Autodesk Inventor part; units mm, degrees
ref_plane "YZ Plane" through (0, 0, 0) normal (1, 0, 0) x (0, 1, 0)
ref_plane "XZ Plane" through (0, 0, 0) normal (0, 1, 0) x (-1, 0, 0)
ref_plane "XY Plane" through (0, 0, 0) normal (0, 0, 1) x (1, 0, 0)
sketch "Sketch1" plane through (0, 0, 0) normal (0, 1, 0) x (-1, 0, 0)
  line L0 (6.15, 6.15) -> (-6.15, 6.15)
  line L1 (-6.15, 6.15) -> (-6.15, -6.15)
  line L2 (-6.15, -6.15) -> (6.15, -6.15)
  line L3 (6.15, -6.15) -> (6.15, 6.15)
  point P0 (0, 0)
  dimension "d0" = 12.3
  dimension "d1" = 12.3
  dimension "d2" = 6.15
  dimension "d3" = 6.15
extrude "Extrusion1" add sketch "Sketch1" along normal blind 5.5
fillet "Fillet1" radius 3.175 4 edges at (6.15, 2.75, 6.15) (-6.15, 2.75, 6.15) (6.15, 2.75, -6.15) (-6.15, 2.75, -6.15)
sketch "Sketch2" plane through (0, 5.5, 0) normal (0, 1, 0) x (1, 0, 0)
  circle A0 centre (0, 0) radius 4.9967
extrude "Extrusion2" add sketch "Sketch2" along normal blind 0.5
chamfer "Chamfer1" distance 1 angle 45 8 edges at (0, 0, 6.15) (5.2201, 0, 5.2201) (6.15, 0, 0) (5.2201, 0, -5.2201) (0, 0, -6.15) (-5.2201, 0, -5.2201) (-6.15, 0, 0) (-5.2201, 0, 5.2201)
sketch "Sketch3" plane through (0, 0, 0) normal (0, -1, 0) x (1, 0, 0)
  line L0 (-6, -2.5) -> (-3.8, -2.5)
  line L1 (-3.8, -2.5) -> (-3.8, -0.7387)
  line L2 (-3.8, -0.7387) -> (-6, -0.7387)
  line L3 (-6, -0.7387) -> (-6, -2.5)
  point P0 (0, 0)
  dimension "d12" = 2.5
  dimension "d13" = 3.8
  dimension "d16" = 6
extrude "Extrusion3" add sketch "Sketch3" against normal blind 1
mirror "Mirror1" about plane through (0, 0, 0) normal (0, 0, 1) of "Extrusion3"
mirror "Mirror2" about plane through (0, 0, 0) normal (1, 0, 0) of "Extrusion3", "Mirror1"
properties part number "Inductor_SMD_12mm"
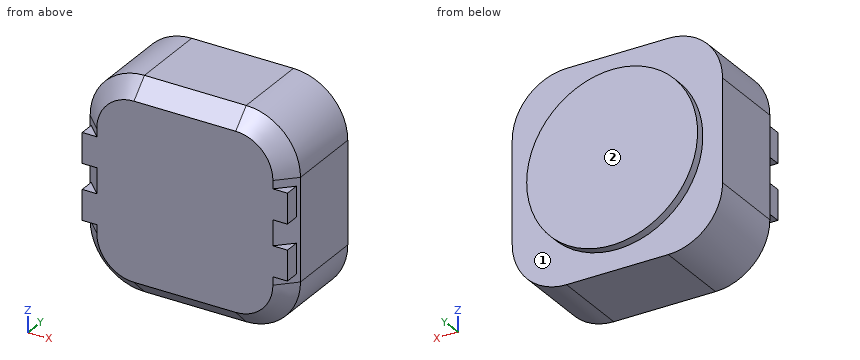
Work out the finished part from the listing and answer in its coordinate system (mm). Face numbers are marked on the shaded views. A direction names the side the tool comes from. Round coordinates to 2 decimals unless told otherwise and drop trailing zeros. Order: outer loops, then holes, each group sorted by start corner. A loop starts at its lowest first (then second) coordinate and runs counter-clockwise, first axis right, second up.
Q1. A cutting plane is placed at C-C, the plane y = 2.2. Determine the outline of the cut face in (x, z) (3 decimals).
Solution:
outline: (-6.15, -2.975) arc R3.175 ccw to (-2.975, -6.15) - (2.975, -6.15) arc R3.175 ccw to (6.15, -2.975) - (6.15, 2.975) arc R3.175 ccw to (2.975, 6.15) - (-2.975, 6.15) arc R3.175 ccw to (-6.15, 2.975) - close
Q2. Find the intervals of material crossed by line 1 along Y through (x, z) = (-3.25, -4.5); line 2 along X through (y, z) = (0.2, -2.25); line 3 along Y through (x, z) = (-5, -4.25), in increasing order.
Solution:
line 1: y = 0 to 5.5
line 2: x = -6 to 6
line 3: y = 0.22 to 5.5
Q3. Given pin 1 Ø0.7 at (y, z) = (0, -2) entering from -X; pin 2 Ø0.9 at (x, y) = (-5.5, 0.5) entering from -Z; pin 3 Ø0.9 at (x, y) = (-5.5, 0.5) entering from +Z; pin 4 Ø4 at (x, z) = (-3, 2.5) entering from -Y, each flat-ended and moving along its own axis, determine where each tip first touches the part or whether it passes through.
Solution:
pin 1: stops at x = -6
pin 2: stops at z = -5.01
pin 3: stops at z = 5.01
pin 4: stops at y = 0
Q4. A cutting plane is placed at A-A, the plane z = 0. Determine the outline of the cut face in (x, y), then the cut area to 3 significant figures.
Solution:
outline: (-6.15, 1) - (-5.15, 0) - (5.15, 0) - (6.15, 1) - (6.15, 5.5) - (5, 5.5) - (5, 6) - (-5, 6) - (-5, 5.5) - (-6.15, 5.5) - close
area: 71.6 mm2
Q5. A tool of negligible diameter and unlimited length cuts with its end or side. For the marked faces 1 and 2, from which of +Z, -Z, +X, -X, +Y, -Y can it reach the whole face along a straight path? Write none if from no direction.
Solution:
face 1: +Y
face 2: +Z, -Z, +X, -X, +Y
Q6. A cutting plane is placed at D-D, the plane z = 1.75. Determine the outline of the cut face in (x, y).
Solution:
outline: (-6.15, 1) - (-6, 0.85) - (-6, 0) - (6, 0) - (6, 0.85) - (6.15, 1) - (6.15, 5.5) - (4.68, 5.5) - (4.68, 6) - (-4.68, 6) - (-4.68, 5.5) - (-6.15, 5.5) - close
Q7. A cutting plane is placed at B-B, the plane x = 0. Determine the outline of the cut face in (y, z).
Solution:
outline: (0, -5.15) - (1, -6.15) - (5.5, -6.15) - (5.5, -5) - (6, -5) - (6, 5) - (5.5, 5) - (5.5, 6.15) - (1, 6.15) - (0, 5.15) - close
